Model file for the job. Use its own axes, mm. A direction names the side the tool comes from. Round coordinates to 2 decimals unless told otherwise and drop trailing zeros. Loops run counter-clockwise (first coordinate to the right, second up) from the corner with the lowest first, then second, coordinate; pieces in that order, holes last. Notation, with made-up numbers: (-3.5, 62.5) -> (32.5, 62.5) arc R9 ccw to (32.5, 73.5) -> close; hole circle Ø1 at (77.25, -22). An arc over 180 degrees is marked (long way). Use a Markdown table: item, result.
from build123d import *

# Parameters (mm, degrees)
F0_R     = 12.7
F0_W     = 2.54
F0_H     = 2.54
F1_DEPTH = 27.94


with BuildPart() as f1:
    # F0 (on Front) → F1 (new body)
    with BuildSketch(Plane.XZ):
        Circle(F0_R)
        with BuildLine():
            ThreePointArc((1.27, 9.4399536545), (6.7351920908, 6.7351920908), (9.4399536545, 1.27))
            Line((9.4399536545, 1.27), (11.43, 1.27))
            Line((11.43, 1.27), (11.43, -1.27))
            Line((11.43, -1.27), (9.4399536545, -1.27))
            ThreePointArc((9.4399536545, -1.27), (6.7351920908, -6.7351920908), (1.27, -9.4399536545))
            Line((1.27, -9.4399536545), (1.27, -11.43))
            Line((1.27, -11.43), (-1.27, -11.43))
            Line((-1.27, -11.43), (-1.27, -9.4399536545))
            ThreePointArc((-1.27, -9.4399536545), (-6.7351920908, -6.7351920908), (-9.4399536545, -1.27))
            Line((-9.4399536545, -1.27), (-11.43, -1.27))
            Line((-11.43, -1.27), (-11.43, 1.27))
            Line((-11.43, 1.27), (-9.4399536545, 1.27))
            ThreePointArc((-9.4399536545, 1.27), (-6.7351920908, 6.7351920908), (-1.27, 9.4399536545))
            Line((-1.27, 9.4399536545), (-1.27, 11.43))
            Line((-1.27, 11.43), (1.27, 11.43))
            Line((1.27, 11.43), (1.27, 9.4399536545))
        make_face(mode=Mode.SUBTRACT)
        with BuildLine():
            ThreePointArc((9.4399536545, -1.27), (9.5037146306, -0.6364222028), (9.525, 0))
            ThreePointArc((9.525, 0), (9.5037146306, 0.6364222028), (9.4399536545, 1.27))
            Line((9.4399536545, 1.27), (1.27, 1.27))
            Line((1.27, 1.27), (1.27, -1.27))
            Line((1.27, -1.27), (9.4399536545, -1.27))
        make_face()
        with BuildLine():
            Line((-1.27, -1.27), (-1.27, 1.27))
            Line((-1.27, 1.27), (-9.4399536545, 1.27))
            ThreePointArc((-9.4399536545, 1.27), (-9.525, 0), (-9.4399536545, -1.27))
            Line((-9.4399536545, -1.27), (-1.27, -1.27))
        make_face()
        with BuildLine():
            Line((1.27, 1.27), (1.27, 9.4399536545))
            ThreePointArc((1.27, 9.4399536545), (0, 9.525), (-1.27, 9.4399536545))
            Line((-1.27, 9.4399536545), (-1.27, 1.27))
            Line((-1.27, 1.27), (1.27, 1.27))
        make_face()
        with BuildLine():
            ThreePointArc((-1.27, -9.4399536545), (0, -9.525), (1.27, -9.4399536545))
            Line((1.27, -9.4399536545), (1.27, -1.27))
            Line((1.27, -1.27), (-1.27, -1.27))
            Line((-1.27, -1.27), (-1.27, -9.4399536545))
        make_face()
        Rectangle(F0_W, F0_H)
        with BuildLine():
            ThreePointArc((-9.4399536545, -1.27), (-9.525, 0), (-9.4399536545, 1.27))
            Line((-9.4399536545, 1.27), (-11.43, 1.27))
            Line((-11.43, 1.27), (-11.43, -1.27))
            Line((-11.43, -1.27), (-9.4399536545, -1.27))
        make_face()
        with BuildLine():
            ThreePointArc((-1.27, 9.4399536545), (0, 9.525), (1.27, 9.4399536545))
            Line((1.27, 9.4399536545), (1.27, 11.43))
            Line((1.27, 11.43), (-1.27, 11.43))
            Line((-1.27, 11.43), (-1.27, 9.4399536545))
        make_face()
        with BuildLine():
            Line((1.27, -11.43), (1.27, -9.4399536545))
            ThreePointArc((1.27, -9.4399536545), (0, -9.525), (-1.27, -9.4399536545))
            Line((-1.27, -9.4399536545), (-1.27, -11.43))
            Line((-1.27, -11.43), (1.27, -11.43))
        make_face()
        with BuildLine():
            ThreePointArc((9.4399536545, 1.27), (9.5037146306, 0.6364222028), (9.525, 0))
            ThreePointArc((9.525, 0), (9.5037146306, -0.6364222028), (9.4399536545, -1.27))
            Line((9.4399536545, -1.27), (11.43, -1.27))
            Line((11.43, -1.27), (11.43, 1.27))
            Line((11.43, 1.27), (9.4399536545, 1.27))
        make_face()
    extrude(amount=F1_DEPTH)


solid = f1.part
Q1. Band-saw the part on B-B, the plane z = 2.5. Give the cut face in (x, y), plus the area to 3 significant figures.
Results list:
| item | result |
|---|---|
| outline | (-12.45, -27.94) -> (-9.19, -27.94) -> (-9.19, 0) -> (-12.45, 0) -> close; (-1.27, -27.94) -> (1.27, -27.94) -> (1.27, 0) -> (-1.27, 0) -> close; (9.19, -27.94) -> (12.45, -27.94) -> (12.45, 0) -> (9.19, 0) -> close |
| area | 253 mm² |
Q2. Pull direction X, two halves, no side cores. Call faces 1 (the face through (0, 0, 0)), 2 (the face through (6.67, -13.77, 6.8)), 3 (the face through (-2.75, -13.77, -12.4)), 4 (the face through (6.8, -13.77, -6.67)): released by +X, released by -X, zero draft, split by the parting line, or undercut.
Results list:
| item | result |
|---|---|
| face 1 | zero draft |
| face 2 | undercut |
| face 3 | split by the parting line |
| face 4 | undercut |
Q3. Band-saw the part on C-C, the plane x = 6. Give the cut face in (y, z), plus the area to 3 significant figures.
Results list:
| item | result |
|---|---|
| outline | (-27.94, -11.19) -> (0, -11.19) -> (0, -7.4) -> (-27.94, -7.4) -> close; (-27.94, -1.27) -> (0, -1.27) -> (0, 1.27) -> (-27.94, 1.27) -> close; (-27.94, 7.4) -> (0, 7.4) -> (0, 11.19) -> (-27.94, 11.19) -> close |
| area | 283 mm² |
Q4. Drill centre lines: L1, parallel to X at y = -3.5, z = -1.75; L2, parallel to X at y = -24, z = 5.25; L3, parallel to Z at x = -4.5, y = -18.5. Where is each one in solid material? Low to high. Write a range as from..to.
Results list:
| item | result |
|---|---|
| L1 | x = -12.58..-9.36, -1.27..1.27, 9.36..12.58 |
| L2 | x = -11.56..-7.95, -1.27..1.27, 7.95..11.56 |
| L3 | z = -11.88..-8.39, -1.27..1.27, 8.39..11.88 |
Q5. Flat gauge pins, fed straight in: pin 1 (1 mm diameter, centred on x = -4, y = -23.5, fed in from -Z); pin 2 (6.5 mm diameter, centred on y = -20, z = 5, fed in from -X); pin 3 (1.5 mm diameter, centred on x = -3, y = -22.5, fed in from +Z). Where does each tip first touch, or does it go through?
Results list:
| item | result |
|---|---|
| pin 1 | stops at z = -12.21 |
| pin 2 | stops at x = -12.58 |
| pin 3 | stops at z = 12.5 |
Q6. Band-saw the part on A-A, the plane y = -17.25. Give the cut face in (x, z) (3 decimals).
Results list:
| item | result |
|---|---|
| outline | circle Ø25.4 at (0, 0); hole (-9.44, -1.27) arc R9.525 ccw to (-1.27, -9.44) -> (-1.27, -1.27) -> close; hole (-9.44, 1.27) -> (-1.27, 1.27) -> (-1.27, 9.44) arc R9.525 ccw to start; hole (1.27, -9.44) arc R9.525 ccw to (9.44, -1.27) -> (1.27, -1.27) -> close; hole (1.27, 1.27) -> (9.44, 1.27) arc R9.525 ccw to (1.27, 9.44) -> close |
Q7. Tool access for faces 5 (the face through (0, -27.94, 0)), 6 (the face through (5, -14, -1.27)): list every direction of +Z, -Z, +X, -X, +Y, -Y with a clear straight run to the whole face (end or side of a thin tool).
Results list:
| item | result |
|---|---|
| face 5 | +Z, -Z, +X, -X, -Y |
| face 6 | +Y, -Y |
